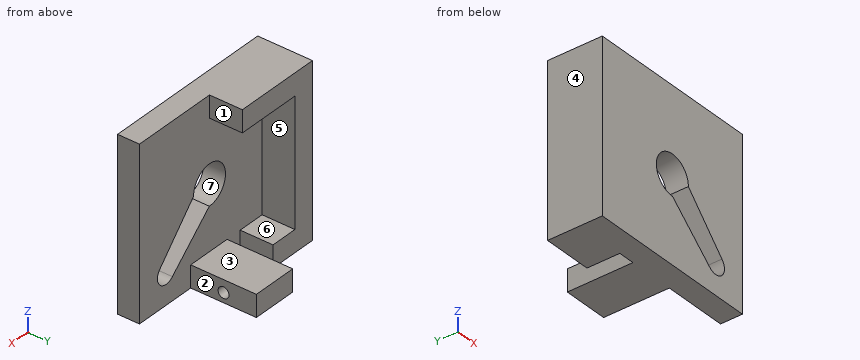
```python
from build123d import *

# Parameters (mm, degrees)
SKETCH1_W           = 32
SKETCH1_H           = 31
BOSS_EXTRUDE1_DEPTH = 4
BOSS_EXTRUDE2_DEPTH = 6
SKETCH5_W           = 8.3
SKETCH5_H           = 4
BOSS_EXTRUDE3_DEPTH = 12
SKETCH6_R           = 1
CUT_EXTRUDE7_DEPTH  = 5
CUT_EXTRUDE6_DEPTH  = 4


with BuildPart() as part:
    # Sketch1 → Boss-Extrude1 (new body)
    with BuildSketch(Plane(origin=(0, 0, 0), x_dir=(1, 0, 0), z_dir=(0, 1, 0))):
        Rectangle(SKETCH1_W, SKETCH1_H)
    extrude(amount=BOSS_EXTRUDE1_DEPTH)

    # Sketch2 → Boss-Extrude2 (add)
    with BuildSketch(Plane(origin=(0, 4, 0), x_dir=(1, 0, 0), z_dir=(0, 1, 0))):
        Polygon((-16, 15.5), (-16, -15.5), (0, -15.5), (0, -11.5), (-12, -11.5), (-12, 11.5), (-7, 11.5), (-7, 15.5), align=None)
    extrude(amount=BOSS_EXTRUDE2_DEPTH)

    # Sketch5 → Boss-Extrude3 (add)
    with BuildSketch(Plane(origin=(0, 4, 0), x_dir=(1, 0, 0), z_dir=(0, 1, 0))):
        with Locations((0.15, 13.5)):
            Rectangle(SKETCH5_W, SKETCH5_H)
    extrude(amount=BOSS_EXTRUDE3_DEPTH)

    # Sketch6 → Cut-Extrude7 (cut)
    with BuildSketch(Plane(origin=(4.3, 0, 0), x_dir=(0, 0, -1), z_dir=(1, 0, 0))):
        with Locations((13.75, 10)):
            Circle(SKETCH6_R)
    extrude(amount=-CUT_EXTRUDE7_DEPTH, mode=Mode.SUBTRACT)

    # Sketch4 → Cut-Extrude6 (cut)
    with BuildSketch(Plane(origin=(0, 4, 0), x_dir=(0.7071067811864886, 0, -0.7071067811866065), z_dir=(0, 1, 0))):
        with BuildLine():
            Line((14, 2), (2.611512971, 2.55))
            ThreePointArc((2.611512971, 2.55), (3.380423224, 1.376676733), (3.65, 0))
            ThreePointArc((3.65, 0), (3.380423224, -1.376676733), (2.611512971, -2.55))
            Line((2.611512971, -2.55), (14, -2))
            ThreePointArc((14, -2), (15.414213562, -1.414213562), (16, 0))
            ThreePointArc((16, 0), (15.414213562, 1.414213562), (14, 2))
        make_face()
        with BuildLine():
            ThreePointArc((3.65, 0), (3.380423224, 1.376676733), (2.611512971, 2.55))
            ThreePointArc((2.611512971, 2.55), (-3.65, 0), (2.611512971, -2.55))
            ThreePointArc((2.611512971, -2.55), (3.380423224, -1.376676733), (3.65, 0))
        make_face()
    extrude(amount=-CUT_EXTRUDE6_DEPTH, mode=Mode.SUBTRACT)


solid = part.part
```
The model under review builds one solid part; all positions refer to its coordinate system, in mm. Face numbers are marked on the shaded views. A direction names the side the tool comes from. Coordinates: 2 decimals unless noted, no trailing zeros. Order: outer loops, then holes, each group sorted by start corner. A loop starts at its lowest first (then second) coordinate and runs counter-clockwise, first axis right, second up. Notation, with made-up numbers: M 53.5,48 L 76.5,48 A11 ccw 76.5,67 Z; hole C -11.5,4.5 d1. An arc over 180 degrees is marked long. One line per question, with ' | ' between items.
(1) Add section D-D, the plane x = -8. Write out the cut boundary in (y, z).
Geometry results:
outline: M 0,-15.5 L 10,-15.5 L 10,-11.5 L 4,-11.5 L 4,11.5 L 10,11.5 L 10,15.5 L 0,15.5 Z
(2) The part is to be moulded in two halves that separate along X. For the marked faces 4, 5, 6 and 7, say which applies: +X half, -X half, draft (parallel to the pull), parting line (faces both ways), or undercut.
Geometry results:
face 4: -X half | face 5: +X half | face 6: draft | face 7: undercut
(3) Add section B-B, the plane z = -13.75. Write out the cut boundary in (x, y).
Geometry results:
outline: M -16,0 L 16,0 L 16,4 L 4.3,4 L 4.3,9 L -0.7,9 L -0.7,11 L 4.3,11 L 4.3,16 L -4,16 L -4,4 L -7,4 L -7,10 L -16,10 Z
(4) For probe 1 along X at (y, z) = (7.5, -13); probe 2 along X at (y, z) = (2.9, 0); probe 3 along Z at (x, y) = (0, 2.4), list the stretches that pass through material, from the lowest coordinate up. Write a range as from..to.
Geometry results:
probe 1: x = -16..-7, -4..4.3 | probe 2: x = -16..-3.65, 3.65..16 | probe 3: z = -15.5..-3.65, 3.65..15.5
(5) Machinability: for the marked faces 1, 2 and 3, which of the approach directions +Z, -Z, +X, -X, +Y, -Y give a long, thin tool a straight path to every point of the face, cutting with its end or side? Answer none if there is none.
Geometry results:
face 1: +Z, +X, +Y | face 2: +Z, -Z, +X, +Y | face 3: +X, +Y
(6) Add section A-A, the plane y = 7. Write out the cut boundary in (x, z), then the cut area to 3 significant figures.
Geometry results:
outline: M -16,-15.5 L -7,-15.5 L -7,-11.5 L -12,-11.5 L -12,11.5 L 0,11.5 L 0,15.5 L -16,15.5 Z; M -4,-15.5 L 4.3,-15.5 L 4.3,-11.5 L -4,-11.5 Z | area: 225 mm²
(7) Add section C-C, the plane x = 8. Write out the cut boundary in (y, z).
Geometry results:
outline: M 0,-15.5 L 4,-15.5 L 4,-10.87 L 0,-10.87 Z; M 0,-4.84 L 4,-4.84 L 4,15.5 L 0,15.5 Z
(8) Insertion check: pin 1 (3 mm diameter, centred on x = 11, z = -1.5, fed in from +Y); pin 2 (0.6 mm diameter, centred on y = 10, z = -13.5, fed in from +X); pin 3 (4 mm diameter, centred on x = 1, z = 1, fed in from -Y); pin 4 (3 mm diameter, centred on y = 6.5, z = -13, fed in from +X). Each pin has a flat end and moves straight along its axis. Give the tip position at first contact, or say it passes through.
Geometry results:
pin 1: stops at y = 4 | pin 2: stops at x = -0.7 | pin 3: passes through | pin 4: stops at x = 4.3
